from build123d import *

# Parameters (mm, degrees)
F0_W     = 8.2234106958
F0_H     = 7.1954836603
F1_DEPTH = 31.75
F2_W     = 108.9601889253
F2_H     = 20.5585248768
F3_DEPTH = 63.5
F4_W     = 13.2161937654
F4_H     = 5.2864775062
F4_W_2   = 0.5873870105
F5_DEPTH = 25.4


with BuildPart() as f1:
    # F0 (on Front) → F1 (new body, symmetric)
    with BuildSketch(Plane.XZ):
        Polygon((-19.0900564194, 5.2864807658), (-19.0900564194, -19.0548436975), (-19.0900564194, -32.0125594735), (-13.2161900401, -32.0125594735), (18.796371296, -32.0125594735), (18.796371296, -20.5585230142), (10.5729606003, -20.5585230142), (10.5729606003, -13.3630393539), (18.796371296, -13.3630393539), (18.796371296, 5.2864807658), align=None)
        with Locations((14.6846659482, -16.960781184)):
            Rectangle(F0_W, F0_H)
        with BuildLine():
            ThreePointArc((-19.0900564194, -19.0548436975), (-31.1716974247, -27.2697965826), (-35.8305685222, -41.1170497537))
            Line((-35.8305685222, -41.1170497537), (-12.9224974662, -41.1170497537))
            Line((-12.9224974662, -41.1170497537), (-13.2161900401, -32.0125594735))
            Line((-13.2161900401, -32.0125594735), (-19.0900564194, -32.0125594735))
            Line((-19.0900564194, -32.0125594735), (-19.0900564194, -19.0548436975))
        make_face()
    extrude(amount=F1_DEPTH, both=True)

    # F2 (on Front) → F3 (join, symmetric)
    with BuildSketch(Plane.XZ):
        with Locations((18.9432166517, -51.3963121921)):
            Rectangle(F2_W, F2_H)
    extrude(amount=F3_DEPTH, both=True)

    # F4 (on Front) → F5 (join)
    with BuildSketch(Plane.XZ):
        with Locations((23.6423071474, -14.3909677863)):
            Rectangle(F4_W, F4_H)
        Polygon((30.2504040301, -3.5243185703), (30.2504040301, -11.7477290332), (30.8377910405, -11.7477290332), (30.8377910405, -17.0342065394), (30.2504040301, -17.0342065394), (30.2504040301, -25.845002383), (52.8647787869, -25.845002383), (52.8647787869, -3.5243185703), align=None)
        with Locations((30.5440975353, -14.3909677863)):
            Rectangle(F4_W_2, F4_H)
    extrude(amount=F5_DEPTH)


solid = f1.part
Verification items for the finished model (mm, model axes). A direction names the side the tool comes from. Coordinates: 2 decimals unless noted, no trailing zeros. Write each loop counter-clockwise with the first axis right and the second up, starting at its lowest first coordinate (ties: lowest second). Pieces come first, ordered by that corner, then holes. Notation, with made-up numbers: (-37, 49.25) - (22, 49.25) arc R35 ccw to (22, 84.25) - close; hole circle Ø9 at (-40, 28.25). An arc over 180 degrees is marked (long way). Answer as a JSON object with one key per item and string values.
(1) Mould release check, pull along X, two halves, no side actions. Record for faces 1 (the cylindrical face through (-31.045, -0.444, -27.105)), 2 (the flat face through (18.796, 0, -18)), 3 (the flat face through (24, -13, -17.034)), 4 (the flat face through (-3, -31.75, -18)): pulls with the +X half, pulls with the -X half, needs draft (parallel to the pull), parting line crosses it, or undercut.
Report:
{"face 1": "pulls with the -X half", "face 2": "undercut", "face 3": "undercut", "face 4": "needs draft"}
(2) Cross-section at C-C on y = 14.5. Record the cut outline in (x, z).
Report:
{"outline": "(-35.83, -41.12) - (-35.54, -41.12) - (-35.54, -61.68) - (73.42, -61.68) - (73.42, -41.12) - (-12.92, -41.12) - (-13.22, -32.01) - (18.8, -32.01) - (18.8, 5.29) - (-19.09, 5.29) - (-19.09, -19.05) arc R22.91 ccw to start"}
(3) Gauge pin test, flat ends, axial feed: pin 1 Ø19.5 at (y, z) = (-14.5, -5.5) entering from -X; pin 2 Ø6 at (x, z) = (10.5, -17) entering from +Y; pin 3 Ø4 at (y, z) = (-22.5, -16.5) entering from +X. Record the tip position at first contact, or that the pin passes through.
Report:
{"pin 1": "x = -19.09", "pin 2": "y = 31.75", "pin 3": "x = 52.86"}
(4) Tool access check on faces 5 (the flat face through (42, -13, -3.524)), 6 (the flat face through (39, 0, -15)), 7 (the flat face through (24, -13, -11.748)). Record the directions out of +Z, -Z, +X, -X, +Y, -Y that give a thin tool (end or side, any length) a straight path to the whole face; none if there is none.
Report:
{"face 5": "+Z, +X, +Y, -Y", "face 6": "+Z, +X, +Y", "face 7": "+Z, +Y, -Y"}
(5) Thickness scan on line 1 along Z through (x, y) = (-12, 21); line 2 along Z through (x, y) = (28, 27); line 3 along Y through (x, z) = (42, -13). Record the ranges inside material, lowest first.
Report:
{"line 1": "-61.68 to -41.12, -32.01 to 5.29", "line 2": "-61.68 to -41.12", "line 3": "-25.4 to 0"}
(6) Cross-section at B-B on z = -5. Record the cut outline in (x, y).
Report:
{"outline": "(-19.09, -31.75) - (18.8, -31.75) - (18.8, 31.75) - (-19.09, 31.75) - close; (30.25, -25.4) - (52.86, -25.4) - (52.86, 0) - (30.25, 0) - close"}
(7) Cross-section at D-D on z = -15. Record the cut outline in (x, y), plus the area to 3 significant figures.
Report:
{"outline": "(-19.09, -31.75) - (18.8, -31.75) - (18.8, -25.4) - (52.86, -25.4) - (52.86, 0) - (18.8, 0) - (18.8, 31.75) - (-19.09, 31.75) - close", "area": "3,270 mm^2"}
(8) Cross-section at A-A on x = 9.5. Record the cut outline in (y, z).
Report:
{"outline": "(-63.5, -61.68) - (63.5, -61.68) - (63.5, -41.12) - (-63.5, -41.12) - close; (-31.75, -32.01) - (31.75, -32.01) - (31.75, 5.29) - (-31.75, 5.29) - close"}
